Geometry check sheet. Reference: the model listing, model coordinates, mm. A direction names the side the tool comes from. Round coordinates to 2 decimals unless told otherwise and drop trailing zeros. Loops run counter-clockwise (first coordinate to the right, second up) from the corner with the lowest first, then second, coordinate; pieces in that order, holes last. Notation, with made-up numbers: (-24, 53) -> (-12, 53) arc R21 ccw to (-12, 75) -> close; hole circle Ø3 at (28, 53). An arc over 180 degrees is marked (long way). Use a Markdown table: item, result. Add a question column.
Q1. Sectioned sample at A-A, the plane z = 20. Enter the section's corners in (x, y).
Q2. Release check for a two-part mould opening along Z. For faces 5 (the face through (-41.888, -61.3, 63.664)), 6 (the face through (-50, -24, 43)), 7 (the face through (-17, -22, 0)), 8 (the face through (-13, -52, 31)) record: released by +Z, released by -Z, zero draft, split by the parting line, or undercut.
Q3. Set-up check for faces 1 (the face through (0, -61, 6)), 2 (the face through (-34, -61, 20)), 3 (the face through (-12.162, -53.095, 35.563)), 4 (the face through (-17, -16.684, 64)): record each of +Z, -Z, +X, -X, +Y, -Y from which the full face is reachable in a straight line by a thin tool's end or side.
Q4. Sectioned sample at C-C, the plane x = 6.5. Enter the section's corners in (y, z).
Q5. Gauge pin test, flat ends, axial feed: P1, Ø12, axis at y = 36.5, z = 78, coming from the +X side; P2, Ø1.5, axis at x = 14.5, z = 55, coming from the -Y side; P3, Ø10, axis at x = -9.5, y = -69.5, coming from the +Z side. Record the tip position at first contact, or that the pin passes through.
Q6. Sectioned sample at D-D, the plane z = 36. Enter the section's corners in (x, y).
Q7. Sectioned sample at B-B, the plane y = 7.5. Enter the section's corners in (x, z), then the cut area to 3 significant figures.
Q8. Material ranges on L1, parallel to Z at x = -8.5, y = -77.5; L2, parallel to Y at x = -17, z = 35; L3, parallel to X at y = -35, z = 65.5, recorded low to high.
```python
from build123d import *

# Parameters (mm, degrees)
F0_W      = 50
F0_H      = 88
F1_DEPTH  = 88
F2_W      = 50
F2_H      = 88
F3_DEPTH  = 48
F4_W      = 16
F4_H      = 88
F5_DEPTH  = 48
F7_DEPTH  = 25
F8_R      = 9
F9_DEPTH  = 31
F11_DEPTH = 34


with BuildPart() as f1:
    # F0 (on Top) → F1 (new body)
    with BuildSketch(Plane.XY):
        with Locations((-25, -60.6841130704)):
            Rectangle(F0_W, F0_H)
        with BuildLine():
            Line((0, 58.3158869296), (-50, 58.3158869296))
            Line((-50, 58.3158869296), (-50, -16.6841130704))
            Line((-50, -16.6841130704), (0, -16.6841130704))
            Line((0, -16.6841130704), (0, -4.1841130704))
            ThreePointArc((0, -4.1841130704), (-25, 20.8158869296), (0, 45.8158869296))
            Line((0, 45.8158869296), (0, 58.3158869296))
        make_face()
        with BuildLine():
            ThreePointArc((0, -16.6841130704), (37.5, 20.8158869296), (0, 58.3158869296))
            Line((0, 58.3158869296), (0, 45.8158869296))
            ThreePointArc((0, 45.8158869296), (17.6776695297, 38.4935564593), (25, 20.8158869296))
            ThreePointArc((25, 20.8158869296), (17.6776695297, 3.1382174), (0, -4.1841130704))
            Line((0, -4.1841130704), (0, -16.6841130704))
        make_face()
    extrude(amount=F1_DEPTH)

    # F2 (on face) → F3 (cut)
    with BuildSketch(Plane.XY.offset(88)):
        with Locations((-25, -60.6841130704)):
            Rectangle(F2_W, F2_H)
    extrude(amount=-F3_DEPTH, mode=Mode.SUBTRACT)

    # F4 (on face) → F5 (join)
    with BuildSketch(Plane.XY.offset(40)):
        with Locations((-42, -60.6841130704)):
            Rectangle(F4_W, F4_H)
    extrude(amount=F5_DEPTH)

    # F6 (on face) → F7 (cut)
    with BuildSketch(Plane.YZ.offset(-34)):
        Polygon((-104.6841130704, 88), (-104.6841130704, 40), (-16.6841130704, 88), align=None)
    extrude(amount=-F7_DEPTH, mode=Mode.SUBTRACT)

    # F8 (on face) → F9 (cut)
    with BuildSketch(Plane.XY.offset(40)):
        with Locations((-17, -60.6841130704)):
            Circle(F8_R)
    extrude(amount=-F9_DEPTH, mode=Mode.SUBTRACT)

    # F10 (on face) → F11 (cut)
    with BuildSketch(Plane.YZ):
        with BuildLine():
            Line((-41.6841130704, 31), (-79.6841130704, 31))
            ThreePointArc((-79.6841130704, 31), (-90.6841130704, 20), (-79.6841130704, 9))
            Line((-79.6841130704, 9), (-41.6841130704, 9))
            ThreePointArc((-41.6841130704, 9), (-30.6841130704, 20), (-41.6841130704, 31))
        make_face()
    extrude(amount=-F11_DEPTH, mode=Mode.SUBTRACT)


solid = f1.part
```
Values:
| question | item | result |
|---|---|---|
| 1 | outline | (-50, -104.68) -> (0, -104.68) -> (0, -90.68) -> (-34, -90.68) -> (-34, -30.68) -> (0, -30.68) -> (0, -16.68) arc R37.5 ccw to (0, 58.32) -> (-50, 58.32) -> close; hole circle Ø50 at (0, 20.82) |
| 2 | face 5 | released by +Z |
| 2 | face 6 | zero draft |
| 2 | face 7 | released by -Z |
| 2 | face 8 | undercut |
| 3 | face 1 | +Z, -Z, +X, -Y |
| 3 | face 2 | +X |
| 3 | face 3 | +Z |
| 3 | face 4 | +Z, +X, -Y |
| 4 | outline | (-16.12, 0) -> (-3.32, 0) -> (-3.32, 88) -> (-16.12, 88) -> close; (44.96, 0) -> (57.75, 0) -> (57.75, 88) -> (44.96, 88) -> close |
| 5 | P1 | x = 36.23 |
| 5 | P2 | y = -14.07 |
| 5 | P3 | z = 40 |
| 6 | outline | (-50, -104.68) -> (0, -104.68) -> (0, -16.68) arc R37.5 ccw to (0, 58.32) -> (-50, 58.32) -> close; hole circle Ø18 at (-17, -60.68); hole circle Ø50 at (0, 20.82) |
| 7 | outline | (-50, 0) -> (-21.16, 0) -> (-21.16, 88) -> (-50, 88) -> close; (21.16, 0) -> (35.06, 0) -> (35.06, 88) -> (21.16, 88) -> close |
| 7 | area | 3,760 mm^2 |
| 8 | L1 | 0 to 9, 31 to 40 |
| 8 | L2 | -104.68 to -69.68, -51.68 to 2.49, 39.15 to 58.32 |
| 8 | L3 | -50 to -34 |
